Geometry check sheet. Reference: the model listing, model coordinates, mm. Face numbers are marked on the shaded views. A direction names the side the tool comes from. Give positions to 0.01 mm unless a question says otherwise; leave off trailing zeros. Order: outer loops, then holes, each group sorted by start corner. A loop starts at its lowest first (then second) coordinate and runs counter-clockwise, first axis right, second up. Notation, with made-up numbers: M -10,69 L 32,69 A31 ccw 32,108 Z; hole C 15,75 d8. An arc over 180 degrees is marked long. Answer as CSV lines item,"result".
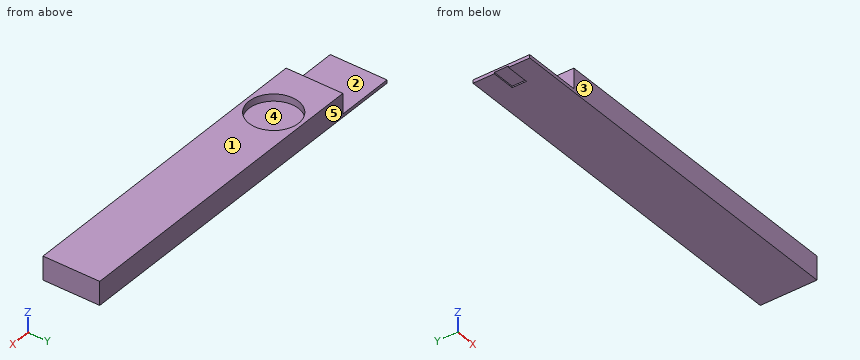
from build123d import *

# Parameters (mm, degrees)
F0_W     = 12.3
F0_H     = 6
F1_DEPTH = 0.7
F3_DEPTH = 5
F4_R     = 5.25
F5_DEPTH = 1.5
F2_W     = 5
F2_H     = 3
F6_DEPTH = 0.3


with BuildPart() as f1:
    # F0 (on Top) → F1 (new body)
    with BuildSketch(Plane.XY):
        with Locations((-33.85, -3)):
            Rectangle(F0_W, F0_H)
        with Locations((-33.85, 3)):
            Rectangle(F0_W, F0_H)
    extrude(amount=F1_DEPTH)

    # F0 (on Top) → F3 (join)
    with BuildSketch(Plane.XY):
        Polygon((40, -6), (40, 6), (-27.7, 6), (-27.7, 0), (-27.7, -6), align=None)
    extrude(amount=F3_DEPTH)

    # F4 (on face) → F5 (cut)
    with BuildSketch(Plane.XY.offset(5)):
        with Locations((-16.35, 0)):
            Circle(F4_R)
    extrude(amount=-F5_DEPTH, mode=Mode.SUBTRACT)

    # F2 (on Top) → F6 (cut)
    with BuildSketch(Plane.XY):
        with Locations((-37.5, 0)):
            Rectangle(F2_W, F2_H)
    extrude(amount=F6_DEPTH, mode=Mode.SUBTRACT)


solid = f1.part
(1) Section check C-C on x = -16.35. Enter the section's corners in (y, z), then the cut area to 4 significant figures.
The answers:
outline,"M -6,0 L 6,0 L 6,5 L 5.25,5 L 5.25,3.5 L -5.25,3.5 L -5.25,5 L -6,5 Z"
area,"44.25 mm2"
(2) Gauge pin test, flat ends, axial feed: P1, Ø5, axis at x = -16.5, y = -2, coming from the +Z side; P2, Ø1.3, axis at y = 2, z = 3.5, coming from the -X side; P3, Ø3, axis at y = -2, z = 1, coming from the -X side; P4, Ø1.5, axis at x = -37.5, y = -0.5, coming from the -Z side. Record the tip position at first contact, or that the pin passes through.
The answers:
P1,"stops at z = 3.5"
P2,"stops at x = -27.7"
P3,"stops at x = -40"
P4,"stops at z = 0.3"
(3) Section check A-A on y = 0. Enter the section's corners in (x, z), then the cut area to 3 significant figures.
The answers:
outline,"M -40,0.3 L -35,0.3 L -35,0 L 40,0 L 40,5 L -11.1,5 L -11.1,3.5 L -21.6,3.5 L -21.6,5 L -27.7,5 L -27.7,0.7 L -40,0.7 Z"
area,"330 mm2"
(4) Section check B-B on z = 4.15. Enter the section's corners in (x, y), then the cut area to 3 significant figures.
The answers:
outline,"M -27.7,-6 L 40,-6 L 40,6 L -27.7,6 Z; hole C -16.35,0 d10.5"
area,"726 mm2"
(5) Tool access check on the marked faces 1 and 2. Record the directions out of +Z, -Z, +X, -X, +Y, -Y that give a thin tool (end or side, any length) a straight path to the whole face; none if there is none.
The answers:
face 1,"+Z, +X, -X, +Y, -Y"
face 2,"+Z, -X, +Y, -Y"
(6) Draft check along Y on the marked faces 3, 4 and 5. Enter one of: +Y half, -Y half, draft (parallel to the pull), parting line (faces both ways), or undercut.
The answers:
face 3,"-Y half"
face 4,"undercut"
face 5,"+Y half"
(7) Material ranges on line 1 (Y direction, x = -16.35, z = 4.2); line 2 (Z direction, x = -30, y = 1); line 3 (X direction, y = 2.75, z = 1), recorded low to high.
The answers:
line 1,"y = -6 to -5.25, 5.25 to 6"
line 2,"z = 0 to 0.7"
line 3,"x = -27.7 to 40"
(8) Section check D-D on y = 3.5. Enter the section's corners in (x, z), then the cut area to 3 significant figures.
The answers:
outline,"M -40,0 L 40,0 L 40,5 L -12.44,5 L -12.44,3.5 L -20.26,3.5 L -20.26,5 L -27.7,5 L -27.7,0.7 L -40,0.7 Z"
area,"335 mm2"
